Geometry: final body of the model. Coordinates: model frame, mm. A direction names the side the tool comes from. Round coordinates to 2 decimals unless told otherwise and drop trailing zeros. Write each loop counter-clockwise with the first axis right and the second up, starting at its lowest first coordinate (ties: lowest second). Pieces come first, ordered by that corner, then holes. Notation, with made-up numbers: (52.25, 1.5) -> (65.25, 1.5) arc R25 cw to (65.25, 34.5) -> close; hole circle Ø1 at (-16.5, 36.25). An arc over 180 degrees is marked (long way). Use one line per item in the form item = value. Start each with the question number.
1. Line query: L1, parallel to X at y = 20, z = 0; L2, parallel to Z at x = -0.5, y = 10; L3, parallel to Z at x = -0.75, y = 18. Output: solid intervals per line, ascending.
2. Pin query (flat end, axial travel): pin 1 Ø3 at (x, y) = (0.5, 26.5) entering from +Z; pin 2 Ø1.5 at (x, y) = (1.5, 11.5) entering from +Z. Return the tip coordinate at first contact, or that it passes through.
3. Cut plane A-A, the plane y = 19. Return the cut outline in (x, z).
4. Reachability of faces 1 (the face through (-1.52, 22.13, 1.66)), 2 (the face through (-0.9, 21.87, -2.86)) from +Z, -Z, +X, -X, +Y, -Y: full face, straight path, thin tool, end or side. Return the list, or none.
```python
from build123d import *


with BuildPart() as part:
    # Esquisse1 → Révolution1 (revolve)
    with BuildSketch(Plane.XY, mode=Mode.PRIVATE) as r_volution1_sk:
        with BuildLine():
            Line((3, 31), (3, 13))
            add(Edge.make_bspline(
                [(3, 13), (3, 10.828758266), (1.909740875, 9.139005261), (1, 4.312648173), (1, 1)],
                knots=[0, 0, 0, 0, 0.47748099, 1, 1, 1, 1], degree=3))
            ThreePointArc((1, 1), (0.707106781, 0.292893219), (0, 0))
            Line((0, 0), (0, 0.75))
            ThreePointArc((0, 0.75), (0.176776695, 0.823223305), (0.25, 1))
            add(Edge.make_bspline(
                [(2.25, 13), (2.25, 12.871737196), (2.245787574, 12.606951452), (2.222038955, 12.143851429), (2.166520076, 11.631917095), (2.066483378, 11.10563901), (1.895459566, 10.465643066), (1.614449871, 9.691395741), (1.208823224, 8.54637983), (0.833436633, 7.090662144), (0.520883429, 5.357160432), (0.341470293, 3.671860451), (0.263896436, 2.196984926), (0.25, 1.39355257), (0.25, 1)],
                knots=[0, 0, 0, 0, 0.03125, 0.0625, 0.125, 0.1875, 0.25, 0.375, 0.5, 0.625, 0.75, 0.875, 0.9375, 1, 1, 1, 1], degree=3))
            Line((2.25, 13), (2.25, 31))
            Line((2.25, 31), (3, 31))
        make_face()
    revolve(r_volution1_sk.sketch.rotate(Axis((0, 0, 0), (0, 1, 0)), 90), axis=Axis((0, 0, 0), (0, 1, 0)))


solid = part.part
```
Outcome:
q1.L1 = -3 to -2.25, 2.25 to 3
q1.L2 = -2.47 to -1.65, 1.65 to 2.47
q1.L3 = -2.9 to -2.12, 2.12 to 2.9
q2.pin_1 = 3
q2.pin_2 = 2.82
q3.outline = circle Ø6 at (0, 0); hole circle Ø4.5 at (0, 0)
q4.face_1 = +Y
q4.face_2 = +Y, -Y
